```python
from build123d import *

# Parameters (mm, degrees)
F0_W        = 80
F0_H        = 80
F1_DEPTH    = 300
F2_R        = 6
F3_W        = 80
F3_H        = 80
F4_DEPTH    = 100
F5_T1_DEPTH = 115


# Not quite as in the source:
# - a fillet or chamfer that OpenCascade refuses, or shapes differently, is made with other operations: its cross-section is extruded or revolved along the edge and cut away or added


with BuildPart() as f1:
    # F0 (on Top) → F1 (new body)
    with BuildSketch(Plane.XY):
        with Locations((-40, 40)):
            Rectangle(F0_W, F0_H)
    extrude(amount=F1_DEPTH)

    # F2
    f2_edges = [f1.edges().sort_by_distance(p)[0] for p in [
        (-80, 80, 150),
        (-80, 0, 150),
        (0, 0, 150),
        (0, 80, 150),
    ]]
    fillet(f2_edges, radius=F2_R)

    # F3 (on Right) → F4 (join)
    with BuildSketch(Plane.YZ):
        with Locations((40, 40)):
            Rectangle(F3_W, F3_H)
    extrude(amount=F4_DEPTH)

    # F5: fillet of radius 6 on 4 edges, made by hand

    # F5_s2 → F5_t1 (cut)
    with BuildSketch(Plane.YZ):
        with BuildLine():
            ThreePointArc((0, 74), (1.7573593129, 78.2426406871), (6, 80))
            Line((6, 80), (0, 80))
            Line((0, 80), (0, 74))
        make_face()
        with BuildLine():
            ThreePointArc((80, 74), (78.2426406871, 78.2426406871), (74, 80))
            Line((74, 80), (80, 80))
            Line((80, 80), (80, 74))
        make_face()
        with BuildLine():
            ThreePointArc((6, 0), (1.7573593129, 1.7573593129), (0, 6))
            Line((0, 6), (0, 0))
            Line((0, 0), (6, 0))
        make_face()
        with BuildLine():
            ThreePointArc((74, 0), (78.2426406871, 1.7573593129), (80, 6))
            Line((80, 6), (80, 0))
            Line((80, 0), (74, 0))
        make_face()
    extrude(amount=F5_T1_DEPTH, mode=Mode.SUBTRACT)


solid = f1.part
```
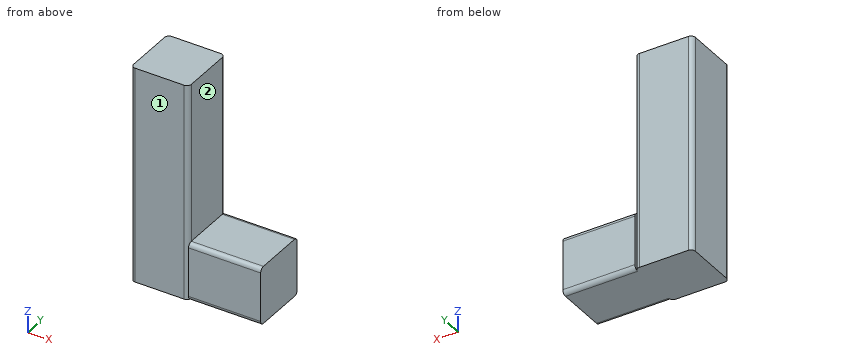
The model under review builds one solid part; all positions refer to its coordinate system, in mm. Face numbers are marked on the shaded views. A direction names the side the tool comes from. Round coordinates to 2 decimals unless told otherwise and drop trailing zeros. Write each loop counter-clockwise with the first axis right and the second up, starting at its lowest first coordinate (ties: lowest second). Pieces come first, ordered by that corner, then holes. Notation, with made-up numbers: (71, 1.5) -> (85, 1.5) arc R16 ccw to (85, 24.5) -> close; hole circle Ø11 at (33.5, -35.75). An arc over 180 degrees is marked (long way). Use CSV: the item, a comma, the result in double quotes.
Q1. To check wall thickness, follow probe 1 along Z at (x, y) = (29, 35.5); probe 2 along X at (y, z) = (61.5, 167.5); probe 3 along Z at (x, y) = (12.5, 75). State the ranges of each line that lie inside material, in increasing order. Write a range as [from, to].
Checks:
probe 1,"[0, 80]"
probe 2,"[-80, 0]"
probe 3,"[0.08, 79.92]"
Q2. Consider section A-A (z = 101). Give the boundary of the cut face in (x, y).
Checks:
outline,"(-80, 6) arc R6 ccw to (-74, 0) -> (-6, 0) arc R6 ccw to (0, 6) -> (0, 74) arc R6 ccw to (-6, 80) -> (-74, 80) arc R6 ccw to (-80, 74) -> close"
Q3. For the marked faces 1 and 2, list the 3-axis set-ups (+Z, -Z, +X, -X, +Y, -Y) from which the entire face can be reached by the end or side of a thin tool; tool diameter is ignored.
Checks:
face 1,"+Z, -Z, +X, -X, -Y"
face 2,"+Z, +X, +Y, -Y"
Q4. For pin 1 Ø5 at (x, y) = (66.5, 8.5) entering from +Z; pin 2 Ø5 at (y, z) = (78.5, 40) entering from -X; pin 3 Ø3 at (y, z) = (4, 22) entering from -X, all flat-tipped, find the tip position at first contact; note any pin that passes through.
Checks:
pin 1,"z = 80"
pin 2,"x = -79.66"
pin 3,"x = -79.98"
Q5. Consider section C-C (y = 17.5). Give the boundary of the cut face in (x, z).
Checks:
outline,"(-80, 0) -> (100, 0) -> (100, 80) -> (0, 80) -> (0, 300) -> (-80, 300) -> close"
Q6. Consider section B-B (x = 59). Give the boundary of the cut face in (y, z), then the cut area to 3 significant figures.
Checks:
outline,"(0, 6) arc R6 ccw to (6, 0) -> (74, 0) arc R6 ccw to (80, 6) -> (80, 74) arc R6 ccw to (74, 80) -> (6, 80) arc R6 ccw to (0, 74) -> close"
area,"6,370 mm²"
